Source: CAD feature listing. Evaluate the final solid. Frame: model axes, mm. Round coordinates to 2 decimals unless told otherwise and drop trailing zeros. Write each loop counter-clockwise with the first axis right and the second up, starting at its lowest first coordinate (ties: lowest second). Pieces come first, ordered by that corner, then holes. Notation, with made-up numbers: (-6, 46) -> (6, 46) arc R31 ccw to (6, 70) -> close; hole circle Ø3 at (-27, 75.25). An arc over 180 degrees is marked (long way). Put each result on its own line as item: value.
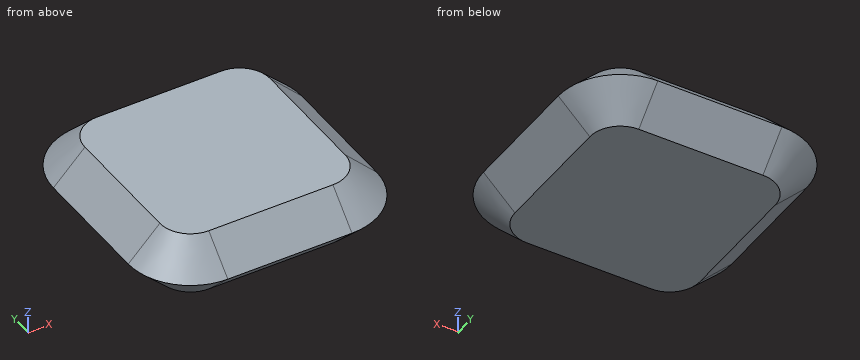
```python
from build123d import *

# Parameters (mm, degrees)
F1_DEPTH = 25.4
F2_SIZE  = 12.69999


# Not quite as in the source:
# - a fillet or chamfer is up to 0.001 mm smaller than in the source, because OpenCascade refuses the exact size


with BuildPart() as f1:
    # F0 (on Top) → F1 (new body)
    with BuildSketch(Plane.XY):
        with BuildLine():
            ThreePointArc((50, 25), (42.6776695297, 42.6776695297), (25, 50))
            Line((25, 50), (-25, 50))
            ThreePointArc((-25, 50), (-42.6776695297, 42.6776695297), (-50, 25))
            Line((-50, 25), (-50, -25))
            ThreePointArc((-50, -25), (-42.6776695297, -42.6776695297), (-25, -50))
            Line((-25, -50), (25, -50))
            ThreePointArc((25, -50), (42.6776695297, -42.6776695297), (50, -25))
            Line((50, -25), (50, 25))
        make_face()
    extrude(amount=F1_DEPTH)

    # F2 (size 12.7 in the source; OpenCascade refuses exactly that, so slightly less here)
    f2_edges = [f1.edges().sort_by_distance(p)[0] for p in [
        (42.67767, 42.67767, 25.4),
        (0, 50, 25.4),
        (-42.67767, 42.67767, 25.4),
        (-50, 0, 25.4),
        (-42.67767, -42.67767, 25.4),
        (0, -50, 25.4),
        (42.67767, -42.67767, 25.4),
        (50, 0, 25.4),
        (42.67767, 42.67767, 0),
        (0, 50, 0),
        (-42.67767, 42.67767, 0),
        (-50, 0, 0),
        (-42.67767, -42.67767, 0),
        (0, -50, 0),
        (42.67767, -42.67767, 0),
        (50, 0, 0),
    ]]
    chamfer(f2_edges, length=F2_SIZE)


solid = f1.part
```
Q1. Pin query (flat end, axial travel): pin 1 (3 mm diameter, centred on y = -23.5, z = 20, fed in from +X); pin 2 (10 mm diameter, centred on x = -2.5, z = 7, fed in from -Y); pin 3 (1 mm diameter, centred on x = -40, y = -20.5, fed in from +Z). Return the tip coordinate at first contact, or that it passes through.
Ans:
pin 1: stops at x = 44.2
pin 2: stops at y = -49.3
pin 3: stops at z = 23.2
Q2. Cut plane A-A on z = 17.5. Output: boundary loops of the cut face in (x, y), and give its area (3 significant figures).
Ans:
outline: (-45.2, -25) arc R20.2 ccw to (-25, -45.2) -> (25, -45.2) arc R20.2 ccw to (45.2, -25) -> (45.2, 25) arc R20.2 ccw to (25, 45.2) -> (-25, 45.2) arc R20.2 ccw to (-45.2, 25) -> close
area: 7,820 mm^2
Q3. Material intervals for line 1 (Y direction, x = 40.5, z = 9.75); line 2 (X direction, y = -38, z = 14.75); line 3 (Z direction, x = 42, y = -20), sorted ascending. Write a range as [from, to].
Ans:
line 1: y = [-40.68, 40.68]
line 2: x = [-43.91, 43.91]
line 3: z = [4.7, 20.7]
